Model file for the job. Use its own axes, mm. A direction names the side the tool comes from. Coordinates: 2 decimals unless noted, no trailing zeros. Order: outer loops, then holes, each group sorted by start corner. A loop starts at its lowest first (then second) coordinate and runs counter-clockwise, first axis right, second up. Notation, with made-up numbers: (1, 21.25) -> (26, 21.25) arc R17 ccw to (26, 45.25) -> close; hole circle Ø3 at (47.5, -40). An arc over 180 degrees is marked (long way). Return JSON: item names as keys, results as strings. Group by question number.
1) Cut at A-A (y = 1.65). State how many separate pieces and enclosed holes the cut face has, and give its area (3 significant figures).
2) Which spindle directions (+Z, -Z, +X, -X, +Y, -Y) get a long thin tool onto all of the face, cutting with end or side? Do faces 5 (the flat face through (6, 1, 0)), 6 (the flat face through (6, 1, -8.89)). Say none if no direction does.
3) Flat gauge pin, fed straight in: pin 1 (1 mm diameter, centred on x = 11, z = -2, fed in from +Y). Where does the tip first touch, or does it go through?
4) Cut at C-C (z = -8.25). Write the cut outline in (x, y) (3 decimals).
5) Pull direction X, two halves, no side cores. Call faces 1 (the flat face through (12.065, 1, -5)), 2 (the flat face through (0, 1, -5)), 3 (the flat face through (0.635, 1, -5)), 4 (the flat face through (6.4, 2.543, -5.3)): +X half, -X half, draft (parallel to the pull), parting line (faces both ways), or undercut.
6) Cut at D-D (x = 10.5). Write the cut outline in (y, z) (3 decimals), and give its area (3 significant figures).
7) Probe line 1 (Z direction, x = 3.5, y = 0.9) (3 decimals); line 2 (X direction, y = 1.45, z = -7.5) (3 decimals); line 3 (X direction, y = 1.3, z = -4.5) (3 decimals). List the from-to ranges inside material, lowest first.
from build123d import *

# Parameters (mm, degrees)
SKETCH1_W           = 12.7
SKETCH1_H           = 9.525
BOSS_EXTRUDE1_DEPTH = 2.54
FILLET1_R           = 0.635
SHELL1_START        = 0.635
SHELL1_OUTLINE_W    = 1.905
SHELL1_OUTLINE_H    = 8.255
SHELL1_DEPTH        = 11.43
SKETCH2_R           = 2.54
BOSS_EXTRUDE2_DEPTH = 1.905
BOSS_EXTRUDE3_DEPTH = 0.00254


# Read off the part's stored shape, not the designer's step: Shell1
with BuildPart() as part:
    # Sketch1 → Boss-Extrude1 (new body)
    with BuildSketch(Plane(origin=(0, 0, 0), x_dir=(1, 0, 0), z_dir=(0, 1, 0))):
        with Locations((6.35, 4.7625)):
            Rectangle(SKETCH1_W, SKETCH1_H)
    extrude(amount=BOSS_EXTRUDE1_DEPTH)

    # Fillet1
    fillet1_edges = [part.edges().sort_by_distance(p)[0] for p in [
        (0, 1.27, -9.525),
        (12.7, 1.27, -9.525),
        (12.7, 1.27, 0),
        (0, 1.27, 0),
    ]]
    fillet(fillet1_edges, radius=FILLET1_R)

    # Shell1 outline → Shell1 (cut)
    with BuildSketch(Plane.YZ.offset(SHELL1_START)):
        with Locations((0.9525, -4.7625)):
            Rectangle(SHELL1_OUTLINE_W, SHELL1_OUTLINE_H)
    extrude(amount=SHELL1_DEPTH, mode=Mode.SUBTRACT)

    # Sketch2 → Boss-Extrude2 (add)
    with BuildSketch(Plane(origin=(0, 1.905, 0), x_dir=(-1, 0, 0), z_dir=(0, -1, 0))):
        with Locations(Location((-6.35, 4.7625, 0), (0, 0, 270))):
            Circle(SKETCH2_R)
    extrude(amount=BOSS_EXTRUDE2_DEPTH)

    # Sketch3 → Boss-Extrude3 (add)
    with BuildSketch(Plane(origin=(0, 2.54, 0), x_dir=(1, 0, 0), z_dir=(0, 1, 0))):
        Polygon((3.414346154, 6.477), (4.961141026, 6.477), (4.961141026, 5.907128205), (3.984217949, 5.907128205), (3.984217949, 5.296551282), (4.961141026, 5.296551282), (4.961141026, 4.726679487), (3.984217949, 4.726679487), (3.984217949, 3.302), (3.414346154, 3.302), align=None)
        Polygon((5.871282252, 6.477), (6.752166667, 6.477), (6.752166667, 3.302), (6.182294872, 3.302), (6.182294872, 5.947833333), (5.531012821, 5.947833333), align=None)
        with BuildLine():
            Line((8.339666667, 5.418666667), (7.769794872, 5.418666667))
            add(Edge.make_bspline(
                [(7.769794872, 5.418666667), (7.772256061, 5.461774453), (7.777065076, 5.54600448), (7.796194123, 5.66835129), (7.82182639, 5.783955572), (7.856036054, 5.89241293), (7.899022734, 5.993683952), (7.949680273, 6.088113879), (8.009302856, 6.175205533), (8.076621518, 6.254538911), (8.150493374, 6.325709616), (8.229384771, 6.388814034), (8.31450246, 6.440886212), (8.404291271, 6.483736794), (8.498735915, 6.517972417), (8.598729985, 6.540861702), (8.70340768, 6.55636255), (8.775068039, 6.557718936), (8.811591747, 6.558410256)],
                knots=[0, 0, 0, 0, 1.199038563, 2.342849363, 3.436047546, 4.486744587, 5.497670872, 6.488682221, 7.459191391, 8.424610317, 9.374430501, 10.305433194, 11.225809216, 12.140057399, 13.06607119, 14.010487599, 14.985989317, 16, 16, 16, 16], degree=3))
            add(Edge.make_bspline(
                [(8.811591747, 6.558410256), (8.85642408, 6.557011369), (8.9439473, 6.554280414), (9.071125482, 6.53098446), (9.189895998, 6.492018376), (9.300172515, 6.437572481), (9.401016227, 6.368404679), (9.492410414, 6.285933395), (9.571591168, 6.188428338), (9.639060519, 6.079946535), (9.695119486, 5.965079574), (9.734403276, 5.846302372), (9.760224087, 5.726766795), (9.762978037, 5.646277588), (9.764346154, 5.606291867)],
                knots=[0, 0, 0, 0, 1.075374347, 2.099382735, 3.09057751, 4.06680945, 5.040638231, 6.016817125, 7.011024321, 8.044445721, 9.0776792, 10.070479129, 11.0414456, 12, 12, 12, 12], degree=3))
            add(Edge.make_bspline(
                [(9.764346154, 5.606291867), (9.763813481, 5.582105677), (9.762741343, 5.53342485), (9.755286624, 5.459758812), (9.744103072, 5.384721339), (9.727241001, 5.308376769), (9.706212616, 5.230703702), (9.680702146, 5.151469689), (9.65011785, 5.071123958), (9.614970118, 4.98876223), (9.573038785, 4.904117111), (9.524215575, 4.815919737), (9.467204612, 4.724248345), (9.402694514, 4.62858533), (9.330371972, 4.529081566), (9.249883932, 4.426036789), (9.162157425, 4.319087904), (9.099895456, 4.247598577), (9.067906851, 4.210869191)],
                knots=[0, 0, 0, 0, 0.728284026, 1.46585585, 2.227944881, 3.01186502, 3.81876927, 4.650621989, 5.517437689, 6.406905708, 7.346299482, 8.360816762, 9.441613733, 10.596154504, 11.834900912, 13.145207542, 14.533280747, 16, 16, 16, 16], degree=3))
            Line((9.067906851, 4.210869191), (8.736541667, 3.831166667))
            Line((8.736541667, 3.831166667), (9.805051282, 3.831166667))
            Line((9.805051282, 3.831166667), (9.805051282, 3.302))
            Line((9.805051282, 3.302), (7.688384615, 3.302))
            Line((7.688384615, 3.302), (7.688384615, 3.590752003))
            Line((7.688384615, 3.590752003), (8.62841867, 4.591207732))
            add(Edge.make_bspline(
                [(8.62841867, 4.591207732), (8.655635071, 4.620391337), (8.70834517, 4.676911324), (8.783346208, 4.759916937), (8.851215523, 4.838687284), (8.910545788, 4.914061108), (8.96445058, 4.983593589), (9.010526288, 5.049380524), (9.049194469, 5.110827174), (9.091174264, 5.184921103), (9.131041269, 5.273291298), (9.167621659, 5.375097387), (9.189919938, 5.47240056), (9.192997806, 5.5358054), (9.194474359, 5.566222756)],
                knots=[0, 0, 0, 0, 1.246127091, 2.413378631, 3.493388633, 4.492180848, 5.408488754, 6.240484944, 6.999099869, 7.674939598, 8.898438119, 10.020720584, 11.050475521, 12, 12, 12, 12], degree=3))
            add(Edge.make_bspline(
                [(9.194474359, 5.566222756), (9.193370376, 5.595649202), (9.191231232, 5.652667658), (9.167723774, 5.733776109), (9.131305205, 5.807211531), (9.079986297, 5.870779591), (9.017823027, 5.923017682), (8.945987529, 5.961870906), (8.865065475, 5.984289038), (8.808337572, 5.987094988), (8.779154848, 5.988538462)],
                knots=[0, 0, 0, 0, 1.062038974, 2.057870785, 3.028805853, 4.01125022, 4.991535629, 5.949134679, 6.94496649, 8, 8, 8, 8], degree=3))
            add(Edge.make_bspline(
                [(8.779154848, 5.988538462), (8.764078681, 5.988005225), (8.734398824, 5.986955463), (8.690771755, 5.979967483), (8.649257465, 5.967651898), (8.609393876, 5.951150747), (8.571606422, 5.929278353), (8.535990417, 5.902317143), (8.5021706, 5.870952262), (8.470302083, 5.835281784), (8.441297572, 5.79547352), (8.415535872, 5.751891037), (8.394235234, 5.704561389), (8.375481378, 5.654109398), (8.361017507, 5.59999317), (8.350486015, 5.542536583), (8.342479625, 5.481833113), (8.340621377, 5.440105185), (8.339666667, 5.418666667)],
                knots=[0, 0, 0, 0, 0.903469896, 1.778625579, 2.63899355, 3.493148037, 4.358286772, 5.247621495, 6.164656832, 7.118446693, 8.109501108, 9.111810964, 10.146451449, 11.215617525, 12.33435995, 13.498009769, 14.714554818, 16, 16, 16, 16], degree=3))
        make_face()
    extrude(amount=BOSS_EXTRUDE3_DEPTH)


solid = part.part
Answers below:
{
 "1": {"separate pieces": "2", "enclosed holes": "1", "area": "46.5 mm^2"},
 "2": {"face 5": "+Z, +X, -X, +Y, -Y", "face 6": "-Y"},
 "3": {"pin 1": "stops at y = 2.54"},
 "4": {"outline": "(0, 0) -> (0.635, 0) -> (0.635, 1.905) -> (12.065, 1.905) -> (12.065, 0) -> (12.7, 0) -> (12.7, 2.54) -> (0, 2.54) -> close"},
 "5": {"face 1": "undercut", "face 2": "-X half", "face 3": "undercut", "face 4": "draft"},
 "6": {"outline": "(0, -9.525) -> (2.54, -9.525) -> (2.54, 0) -> (0, 0) -> (0, -0.635) -> (1.905, -0.635) -> (1.905, -8.89) -> (0, -8.89) -> close", "area": "8.47 mm^2"},
 "7": {"line 1": "z = -9.525 to -8.89, -0.635 to 0", "line 2": "x = 0 to 0.635, 12.065 to 12.7", "line 3": "x = 0 to 0.635, 3.824 to 8.876, 12.065 to 12.7"}
}
